Here's the drawing with two shaded views (mm, measured from the low corner). I have some questions. Coordinates: 2 decimals unless noted, no trailing zeros. Order: outer loops, then holes, each group sorted by start corner. A loop starts at its lowest first (then second) coordinate and runs counter-clockwise, first axis right, second up. Notation, with made-up numbers: (19, 84.25) -> (39, 84.25) arc R20 ccw to (39, 123.25) -> close; hole circle Ø1 at (-3.5, 62). An arc over 180 degrees is marked (long way). Answer in a Markdown table with one row per item. Add a question column.
1. Imagine slicing it at A-A on x = 21. Write out the boundary of the cut face in (y, z).
2. We'd pull the mould along X, two halves only. Please class the marked faces 1, 2 and 3: pulls with the +X half, pulls with the -X half, needs draft (parallel to the pull), parting line crosses it, or undercut.
3. Imagine slicing it at D-D on z = 39. Write out the boundary of the cut face in (x, y).
4. Imagine slicing it at C-C on z = 21. Write out the boundary of the cut face in (x, y), plus the area to 4 significant figures.
5. Imagine slicing it at B-B on y = 4. State how many separate pieces and enclosed holes the cut face has, plus the area to 3 significant figures.
6. If I drill on line 1 along Z through (x, y) = (21, 10); line 2 along Z through (x, y) = (5, 7) (1 decimal), over which ranges is the centre line in solid material (lowest first)? Write a range as [from, to].
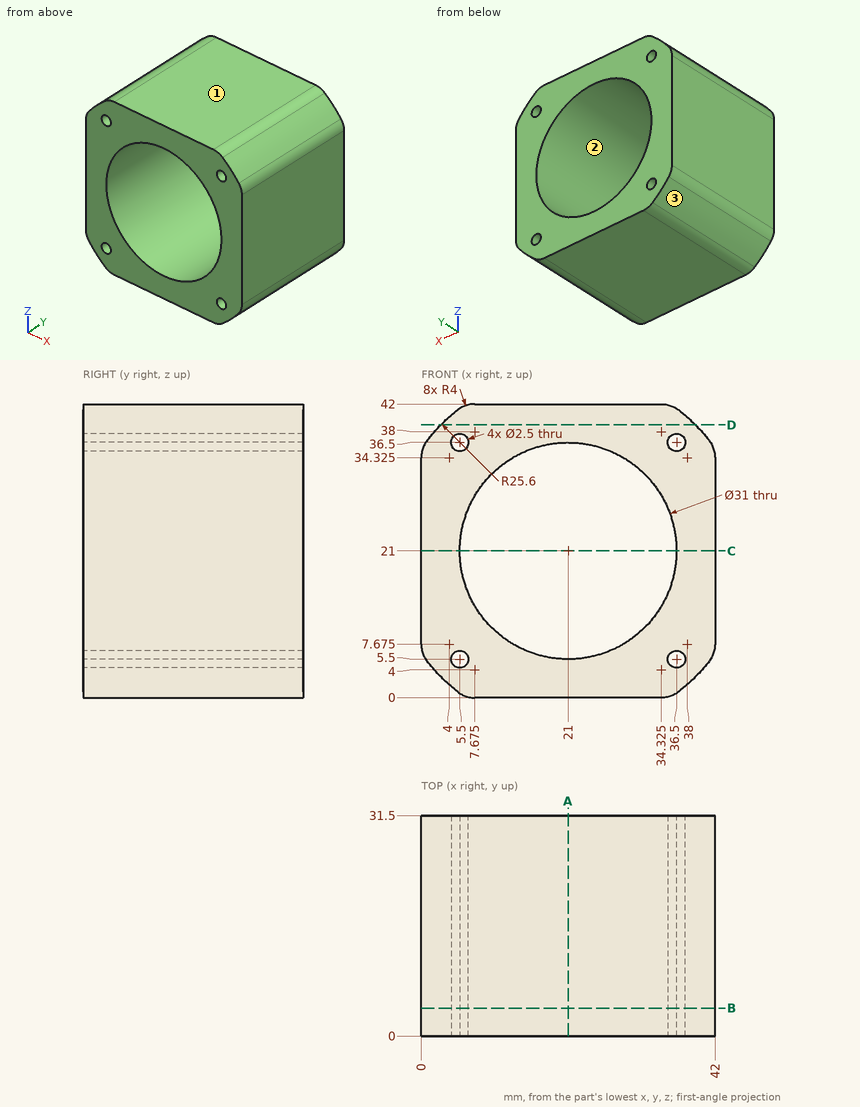
Answers follow:
| question | item | result |
|---|---|---|
| 1 | outline | (0, 0) -> (31.5, 0) -> (31.5, 5.5) -> (0, 5.5) -> close; (0, 36.5) -> (31.5, 36.5) -> (31.5, 42) -> (0, 42) -> close |
| 2 | face 1 | needs draft |
| 2 | face 2 | undercut |
| 2 | face 3 | pulls with the -X half |
| 3 | outline | (2.8, 0) -> (39.2, 0) -> (39.2, 31.5) -> (2.8, 31.5) -> close |
| 4 | outline | (0, 0) -> (5.5, 0) -> (5.5, 31.5) -> (0, 31.5) -> close; (36.5, 0) -> (42, 0) -> (42, 31.5) -> (36.5, 31.5) -> close |
| 4 | area | 346.5 mm² |
| 5 | separate pieces | 1 |
| 5 | enclosed holes | 5 |
| 5 | area | 917 mm² |
| 6 | line 1 | z = [0, 5.5], [36.5, 42] |
| 6 | line 2 | z = [1, 4.4], [6.6, 35.4], [37.6, 41] |
